```python
from build123d import *

# Parameters (mm, degrees)
ESQUISSE1_R             = 4.9
BOSS_EXTRU_1_DEPTH      = 4
ESQUISSE4_R             = 7.5
BOSS_EXTRU_4_DEPTH      = 2
ESQUISSE5_R             = 4.9
BOSS_EXTRU_5_DEPTH      = 4
ENL_V_MAT_EXTRU_1_DEPTH = 15.577379737


with BuildPart() as part:
    # Esquisse1 → Boss.-Extru.1 (new body)
    with BuildSketch(Plane.XY):
        with Locations((0, 1)):
            Circle(ESQUISSE1_R)
    extrude(amount=BOSS_EXTRU_1_DEPTH)

    # Esquisse4 → Boss.-Extru.4 (add)
    with BuildSketch(Plane.XY.offset(4)):
        Circle(ESQUISSE4_R)
    extrude(amount=BOSS_EXTRU_4_DEPTH)

    # Esquisse5 → Boss.-Extru.5 (add)
    with BuildSketch(Plane.XY.offset(6)):
        with Locations((0, -1)):
            Circle(ESQUISSE5_R)
    extrude(amount=BOSS_EXTRU_5_DEPTH)

    # Esquisse6 → Enlèv. mat.-Extru.1 (cut, through all)
    with BuildSketch(Plane.XY.offset(10)):
        with BuildLine():
            Line((-1.5, 2), (1.5, 2))
            ThreePointArc((1.5, 2), (0, -2.5), (-1.5, 2))
        make_face()
    extrude(amount=-ENL_V_MAT_EXTRU_1_DEPTH, mode=Mode.SUBTRACT)


solid = part.part
```
Source: CAD feature listing. Evaluate the final solid. Frame: model axes, mm. A direction names the side the tool comes from. Round coordinates to 2 decimals unless told otherwise and drop trailing zeros. Order: outer loops, then holes, each group sorted by start corner. A loop starts at its lowest first (then second) coordinate and runs counter-clockwise, first axis right, second up. Notation, with made-up numbers: (15.5, 9) -> (43.5, 9) arc R8 ccw to (43.5, 20) -> close; hole circle Ø5 at (10.5, -38). An arc over 180 degrees is marked (long way). Use CSV: the item, a comma, the result in double quotes.
(1) Ray query, L1, parallel to Y at x = 0, z = 2; L2, parallel to Y at x = 0, z = 5.25; L3, parallel to Z at x = 4, y = 2.75. Return the intervals inside material, ascending.
Report:
L1,"-3.9 to -2.5, 2 to 5.9"
L2,"-7.5 to -2.5, 2 to 7.5"
L3,"0 to 6"
(2) First-contact query: pin 1 Ø3 at (y, z) = (3, 4) entering from +X; pin 2 Ø1 at (y, z) = (-0.5, 7) entering from +X. Flat tips, straight axial feed; report the tip coordinate or a pass-through.
Report:
pin 1,"x = 7.35"
pin 2,"x = 4.9"
(3) Access query for faces 1 (the face through (0, -3, 10)), 2 (the face through (3.2, 3.4, 6)), 3 (the face through (4.674, 2.472, 1.972)). Directions: +Z, -Z, +X, -X, +Y, -Y. A direction counts if a zero-diameter tool reaches every point of the face in a straight line with its end or side. Return the directions, or none.
Report:
face 1,"+Z, +X, -X, +Y, -Y"
face 2,"+Z"
face 3,"-Z"
(4) Pull-direction query (Y, two-part tool) for faces 4 (the face through (0, 2, 5)), 5 (the face through (-3.612, 2.312, 7.972)), 6 (the face through (3.2, -3.2, 4)); classes: +Y half, -Y half, draft (parallel to the pull), parting line (faces both ways), or undercut.
Report:
face 4,"undercut"
face 5,"parting line"
face 6,"draft"
(5) Section A-A on x = 0. Return the cut outline in (y, z).
Report:
outline,"(-7.5, 4) -> (-3.9, 4) -> (-3.9, 0) -> (-2.5, 0) -> (-2.5, 10) -> (-5.9, 10) -> (-5.9, 6) -> (-7.5, 6) -> close; (2, 0) -> (5.9, 0) -> (5.9, 4) -> (7.5, 4) -> (7.5, 6) -> (3.9, 6) -> (3.9, 10) -> (2, 10) -> close"
(6) Section C-C on z = 3.5. Return the cut outline in (x, y).
Report:
outline,"circle Ø9.8 at (0, 1); hole (-1.5, 2) arc R2.5 ccw (long way) to (1.5, 2) -> close"
(7) Section B-B on y = -1.5. Return the cut outline in (x, z).
Report:
outline,"(-7.35, 4) -> (-4.21, 4) -> (-4.21, 0) -> (-2, 0) -> (-2, 10) -> (-4.87, 10) -> (-4.87, 6) -> (-7.35, 6) -> close; (2, 0) -> (4.21, 0) -> (4.21, 4) -> (7.35, 4) -> (7.35, 6) -> (4.87, 6) -> (4.87, 10) -> (2, 10) -> close"
(8) Section D-D on y = -3.5. Return the cut outline in (x, z), and give its area (3 significant figures).
Report:
outline,"(-6.63, 4) -> (-1.94, 4) -> (-1.94, 0) -> (1.94, 0) -> (1.94, 4) -> (6.63, 4) -> (6.63, 6) -> (4.21, 6) -> (4.21, 10) -> (-4.21, 10) -> (-4.21, 6) -> (-6.63, 6) -> close"
area,"75.8 mm^2"
